Work out the finished part from the listing and answer in its coordinate system (mm). A direction names the side the tool comes from. Give positions to 0.01 mm unless a question says otherwise; leave off trailing zeros. Loops run counter-clockwise (first coordinate to the right, second up) from the corner with the lowest first, then second, coordinate; pieces in that order, holes last. Notation, with made-up numbers: (53, 86) - (63, 86) arc R17 ccw to (63, 91) - close; hole circle Ø6 at (23.25, -7.5). An arc over 180 degrees is marked (long way). One line per item, written item: value.
from build123d import *

# Parameters (mm, degrees)
LOCATING_HOLE_REACH      = 21.386
LOCATING_HOLE_END_RADIUS = 2.5
LOCATINGHOLES_R          = 0.6


with BuildPart() as part:
    # MainBodyS → MAIN BODY (revolve)
    with BuildSketch(Plane.XY, mode=Mode.PRIVATE) as main_body_sk:
        Polygon((3.45, 0.2), (3.45, 12.7), (3.25, 14.7), (3.25, 17), (3.45, 17), (3.45, 17.6), (3.05, 18), (2, 18), (2, 17.6), (2.5, 17.6), (2.5, 4), (1.1, 4), (1.1, 0), (3.25, 0), align=None)
    revolve(main_body_sk.sketch.rotate(Axis((0, 0, 0), (0, 1, 0)), 90), axis=Axis((0, 0, 0), (0, 1, 0)))

    # LoftedSlotEndS → LOFTED SLOT section 0
    with BuildSketch(Plane(origin=(0, 14.7, 0), x_dir=(-1, 0, 0), z_dir=(0, -1, 0))):
        with BuildLine():
            Line((-1.15, 3.75), (1.15, 3.75))
            Line((1.15, 3.75), (1.15, 3.25))
            Line((1.15, 3.25), (-1.15, 3.25))
            Line((-1.15, 3.25), (-1.15, 3.75))
        make_face()
    # LoftedSlotStartS → LOFTED SLOT section 1
    with BuildSketch(Plane(origin=(0, 0, 0), x_dir=(-1, 0, 0), z_dir=(0, -1, 0))):
        with BuildLine():
            Line((-1.15, 3.45), (1.15, 3.45))
            Line((1.15, 3.45), (1.15, 2.5))
            Line((1.15, 2.5), (-1.15, 2.5))
            Line((-1.15, 2.5), (-1.15, 3.45))
        make_face()
    lofted_slot = loft(mode=Mode.SUBTRACT)

    # LS HM: LOFTED SLOT across plane
    add(lofted_slot.mirror(Plane.XY), mode=Mode.SUBTRACT)

    # LOCATING HOLE: up to this cylinder (the profile starts outside it)
    locating_hole_end = Plane(origin=(0, 5.864986, 0), z_dir=(0, -1, 0)) * Cylinder(LOCATING_HOLE_END_RADIUS, 48.772, mode=Mode.PRIVATE)
    # LocatingHoleS → LOCATING HOLE (cut, up to the surface)
    with BuildSketch(Plane(origin=(0, -0.127219857, 2.493509191), x_dir=(1, 0, 0), z_dir=(0, -0.050954132371911015, 0.9987009944894546)), mode=Mode.PRIVATE) as locating_hole_sk1:
        with Locations(Location((0, 6, 0), (0, 0, 270))):
            Circle(LOCATINGHOLES_R)
    locating_hole_tool1 = extrude(locating_hole_sk1.sketch, amount=-LOCATING_HOLE_REACH, mode=Mode.PRIVATE) - locating_hole_end
    add(locating_hole_tool1.solids().sort_by_distance((0, 5.864986, 2.799234))[0], mode=Mode.SUBTRACT)


solid = part.part
1. Section B-B (y = 15.5) is taken. Write down the section's boundary in (x, z).
Output:
outline: circle Ø6.5 at (0, 0); hole circle Ø5 at (0, 0)
2. Find the intervals of material crossed by line 1 along X through (y, z) = (9, 0); line 2 along X through (y, z) = (2.6, 0); line 3 along Y through (x, z) = (0, 1.25), in increasing order.
Output:
line 1: x = -3.45 to -2.5, 2.5 to 3.45
line 2: x = -3.45 to -1.1, 1.1 to 3.45
line 3: y = 0 to 4
3. The mould has two halves that part along X. Classify faces 4 (the cylindrical face through (0.406, 6.316, 2.635)), 5 (the flat face through (2, 18, -1)), 6 (the conical face through (-3.326, 13.936, -0.073)): released by +X, released by -X, zero draft, split by the parting line, or undercut.
Output:
face 4: undercut
face 5: zero draft
face 6: released by -X
4. Flat-ended cylindrical pins translate along their axes: pin 1 Ø3.5 at (x, z) = (0, 0) entering from +Y; pin 2 Ø2 at (y, z) = (11, 2) entering from -X; pin 3 Ø2 at (x, y) = (-1.5, 2) entering from +Z. Find the tip coordinate at first contact, or state that the pin passes through.
Output:
pin 1: stops at y = 4
pin 2: stops at x = -3.3
pin 3: stops at z = 3.25
5. Section A-A (z = 0) is taken. Write down the section's boundary in (x, y).
Output:
outline: (-3.45, 0.2) - (-3.25, 0) - (-1.1, 0) - (-1.1, 4) - (-2.5, 4) - (-2.5, 17.6) - (-2, 17.6) - (-2, 18) - (-3.05, 18) - (-3.45, 17.6) - (-3.45, 17) - (-3.25, 17) - (-3.25, 14.7) - (-3.45, 12.7) - close; (1.1, 0) - (3.25, 0) - (3.45, 0.2) - (3.45, 12.7) - (3.25, 14.7) - (3.25, 17) - (3.45, 17) - (3.45, 17.6) - (3.05, 18) - (2, 18) - (2, 17.6) - (2.5, 17.6) - (2.5, 4) - (1.1, 4) - close
6. For faces 1 (the cylindrical face through (1.978, 15.866, 2.579)), 2 (the cylindrical face through (1.952, 17.797, 0.434)), 3 (the flat face through (-0.02, 7.25, -2.87)), determine the directions among +Z, -Z, +X, -X, +Y, -Y from which every point of the face is accessible in a straight line to the end or side of a thin tool.
Output:
face 1: none
face 2: +Y
face 3: -Z, -Y
